Source: CAD feature listing. Evaluate the final solid. Frame: model axes, mm. A direction names the side the tool comes from. Coordinates: 2 decimals unless noted, no trailing zeros.
```python
from build123d import *

# Parameters (mm, degrees)
CUT_EXTRUDE1_DEPTH      = 5.5
CUT_EXTRUDE1_DEPTH_BACK = 24.938835821
SKETCH2_W               = 8
SKETCH2_H               = 13
SKETCH2_H_2             = 12
CUT_EXTRUDE2_DEPTH      = 24.938835821
CUT_EXTRUDE2_DEPTH_BACK = 24.938835821
SKETCH3_R               = 1
CUT_EXTRUDE4_START      = -8.000590283
CUT_EXTRUDE4_DEPTH      = 16.001179775
SKETCH6_R               = 0.5
CUT_EXTRUDE5_DEPTH      = 31.03444459
SKETCH7_W               = 8
SKETCH7_H               = 6
CUT_EXTRUDE6_DEPTH      = 27.563957465


with BuildPart() as part:
    # Sketch1 → Revolve1 (revolve)
    with BuildSketch(Plane(origin=(0, 0, 0), x_dir=(0, 0, -1), z_dir=(1, 0, 0))):
        with BuildLine():
            Line((0, 20), (0, -20))
            Line((0, -20), (8, -20))
            add(Edge.make_bspline(
                [(8, 20), (10.604722665, 5.227883705), (8, -20)],
                knots=[0, 0, 0, 1, 1, 1], degree=2))
            Line((8, 20), (0, 20))
        make_face()
    revolve(axis=Axis((0, 20, 0), (0, -1, 0)))

    # Sketch2 → Cut-Extrude1 (cut, two sides: drawn at the far end of the back side and taken through both)
    with BuildSketch(Plane(origin=(0, 0, 0), x_dir=(0, 0, -1), z_dir=(1, 0, 0)).offset(-CUT_EXTRUDE1_DEPTH_BACK)):
        with Locations((0, 13.5)):
            Rectangle(SKETCH2_W, SKETCH2_H)
        with Locations((0, -14)):
            Rectangle(SKETCH2_W, SKETCH2_H_2)
    extrude(amount=CUT_EXTRUDE1_DEPTH + CUT_EXTRUDE1_DEPTH_BACK, mode=Mode.SUBTRACT)

    # Sketch3 → Cut-Extrude2 (cut, two sides: drawn at the far end of the back side and taken through both)
    with BuildSketch(Plane.XY.offset(-CUT_EXTRUDE2_DEPTH_BACK)):
        with Locations(Location((0, 15, 0), (0, 0, 270))):
            Circle(SKETCH3_R)
        with Locations(Location((0.535898385, -17, 0), (0, 0, 90))):
            Circle(SKETCH3_R)
    extrude(amount=CUT_EXTRUDE2_DEPTH + CUT_EXTRUDE2_DEPTH_BACK, mode=Mode.SUBTRACT)

    # Cut-Extrude4: read off the stored shape, not the designer's step
    # Cut-Extrude4 outline → Cut-Extrude4 (cut)
    with BuildSketch(Plane.XY.offset(CUT_EXTRUDE4_START)):
        with BuildLine():
            add(Edge.make_bspline(
                [(-7.68379534, -12.692840328), (-7.471741223, -15.13224481), (-7.218169931, -17.567806686), (-6.92820323, -20)],
                knots=[0.390463737, 0.390463737, 0.390463737, 0.390463737, 1, 1, 1, 1], degree=3))
            Line((-6.92820323, -20), (0.286146459, -20))
            ThreePointArc((0.286146459, -20), (-5.120205239, -17.896724626), (-7.68379534, -12.692840328))
        make_face()
    extrude(amount=CUT_EXTRUDE4_DEPTH, mode=Mode.SUBTRACT)

    # Sketch6 → Cut-Extrude5 (cut, through all)
    with BuildSketch(Plane(origin=(0, 7, 0), x_dir=(1, 0, 0), z_dir=(0, 1, 0))):
        with Locations(Location((-3, 0, 0), (0, 0, 270))):
            Circle(SKETCH6_R)
        with Locations(Location((4, 0, 0), (0, 0, 270))):
            Circle(SKETCH6_R)
    extrude(amount=-CUT_EXTRUDE5_DEPTH, mode=Mode.SUBTRACT)

    # Sketch7 → Cut-Extrude6 (cut, through all)
    with BuildSketch(Plane.ZY.offset(-5.5)):
        with Locations((0, -17)):
            Rectangle(SKETCH7_W, SKETCH7_H)
    extrude(amount=-CUT_EXTRUDE6_DEPTH, mode=Mode.SUBTRACT)


solid = part.part
```
1. Section query A-A on y = 15. Count the separate pieces of the cut face and the enclosed holes in it, plus the area to 3 significant figures.
Findings:
separate pieces: 3
enclosed holes: 0
area: 108 mm2
2. Pin query (flat end, axial travel): P1, Ø6, axis at x = -6, y = -8.5, coming from the +Z side; P2, Ø6, axis at y = 12, z = 0.5, coming from the -X side; P3, Ø8, axis at y = -9, z = -5.5, coming from the +X side; P4, Ø1.6, axis at x = 0, y = 15, coming from the +Z side. Return the tip coordinate at first contact, or that it passes through.
Findings:
P1: stops at z = 8.45
P2: stops at x = 5.5
P3: stops at x = 8.83
P4: passes through
3. Access query for faces 4 (the face through (0, -14, -4)), 5 (the face through (3, -20, -6)), 6 (the face through (-2, 7, 0)). Directions: +Z, -Z, +X, -X, +Y, -Y. A direction counts if a zero-diameter tool reaches every point of the face in a straight line with its end or side. Return the directions, or none.
Findings:
face 4: -X, -Y
face 5: +Z, -Z, +X, -X, -Y
face 6: -X, +Y
4. Ray query, line 1 (X direction, y = 2.5, z = 0); line 2 (Y direction, x = 0, z = -5.55); line 3 (X direction, y = -4.5, z = 0). Return the intervals inside material, ascending.
Findings:
line 1: x = -9.3 to -3.5, -2.5 to 3.5, 4.5 to 9.3
line 2: y = -19.99 to -17.84, -16.16 to 14, 16 to 20
line 3: x = -9.15 to -3.5, -2.5 to 3.5, 4.5 to 9.15
5. Draft query along X for faces 1 (the face through (-2.821, -19.372, -5.584)), 2 (the face through (0, 14, -6)), 3 (the face through (3, -20, 6)). Return one class per face: released by +X, released by -X, zero draft, split by the parting line, or undercut.
Findings:
face 1: released by -X
face 2: undercut
face 3: zero draft
